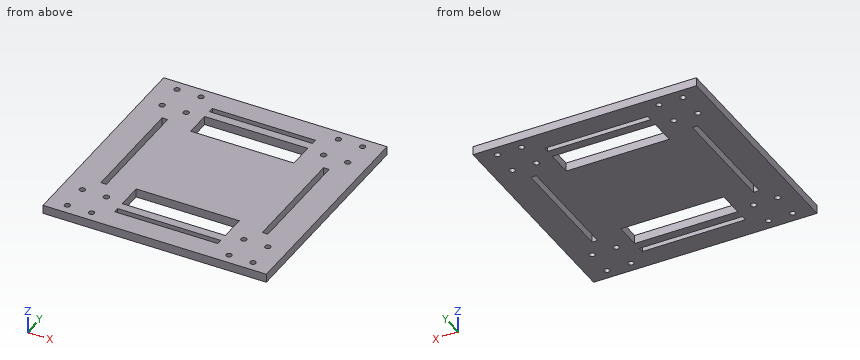
```python
from build123d import *

# Parameters (mm, degrees)
SKETCH_1_W          = 130
SKETCH_1_H          = 130
EXTRUDE_1_DEPTH     = 5
SKETCH_2_R          = 1.65
CUT_EXTRUDE_1_DEPTH = 5
SKETCH_3_W          = 3.2
SKETCH_3_H          = 66
SKETCH_3_W_2        = 60
SKETCH_3_H_2        = 3.2
CUT_EXTRUDE_2_DEPTH = 10
SKETCH_4_W          = 60
SKETCH_4_H          = 15
CUT_EXTRUDE_3_DEPTH = 10


with BuildPart() as part:
    # 草图1 → 凸台-拉伸1 (new body)
    with BuildSketch(Plane.XY):
        Rectangle(SKETCH_1_W, SKETCH_1_H)
    extrude(amount=EXTRUDE_1_DEPTH)

    # 草图2 → 切除-拉伸1 (cut)
    with BuildSketch(Plane.XY.offset(5)):
        with Locations((-54, 59)):
            Circle(SKETCH_2_R)
        with Locations((-40, 59)):
            Circle(SKETCH_2_R)
        with Locations((-40, 43)):
            Circle(SKETCH_2_R)
        with Locations((-54, 43)):
            Circle(SKETCH_2_R)
        with Locations((40, 59)):
            Circle(SKETCH_2_R)
        with Locations((54, 59)):
            Circle(SKETCH_2_R)
        with Locations((54, 43)):
            Circle(SKETCH_2_R)
        with Locations((40, 43)):
            Circle(SKETCH_2_R)
        with Locations((40, -43)):
            Circle(SKETCH_2_R)
        with Locations((54, -43)):
            Circle(SKETCH_2_R)
        with Locations((54, -59)):
            Circle(SKETCH_2_R)
        with Locations((40, -59)):
            Circle(SKETCH_2_R)
        with Locations((-54, -43)):
            Circle(SKETCH_2_R)
        with Locations((-40, -43)):
            Circle(SKETCH_2_R)
        with Locations((-40, -59)):
            Circle(SKETCH_2_R)
        with Locations((-54, -59)):
            Circle(SKETCH_2_R)
    extrude(amount=-CUT_EXTRUDE_1_DEPTH, mode=Mode.SUBTRACT)

    # 草图3 → 切除-拉伸2 (cut)
    with BuildSketch(Plane.XY.offset(5)):
        with Locations((47, 0)):
            Rectangle(SKETCH_3_W, SKETCH_3_H)
        with Locations((-47, 0)):
            Rectangle(SKETCH_3_W, SKETCH_3_H)
        with Locations((0, -51)):
            Rectangle(SKETCH_3_W_2, SKETCH_3_H_2)
        with Locations((0, 51)):
            Rectangle(SKETCH_3_W_2, SKETCH_3_H_2)
    extrude(amount=-CUT_EXTRUDE_2_DEPTH, mode=Mode.SUBTRACT)

    # 草图4 → 切除-拉伸3 (cut)
    with BuildSketch(Plane(origin=(0, 0, 0), x_dir=(-1, 0, 0), z_dir=(0, 0, -1))):
        with Locations((0, 36.9)):
            Rectangle(SKETCH_4_W, SKETCH_4_H)
        with Locations((0, -36.9)):
            Rectangle(SKETCH_4_W, SKETCH_4_H)
    extrude(amount=-CUT_EXTRUDE_3_DEPTH, mode=Mode.SUBTRACT)


solid = part.part
```
Read the model definition and answer for the solid it produces. Units are mm, in the model's axes. Coordinates: 2 decimals unless noted, no trailing zeros. Loops run counter-clockwise (first coordinate to the right, second up) from the corner with the lowest first, then second, coordinate; pieces in that order, holes last. Notation, with made-up numbers: (36.25, 84) -> (77.25, 84) arc R16 cw to (77.25, 115) -> close; hole circle Ø8 at (13.5, 84.25). An arc over 180 degrees is marked (long way). Return JSON: item names as keys, results as strings.
Item 1: Find section B-B (y = 6.5). Determine the outline of the cut face in (x, z).
Answers:
{"outline": "(-65, 0) -> (-48.6, 0) -> (-48.6, 5) -> (-65, 5) -> close; (-45.4, 0) -> (45.4, 0) -> (45.4, 5) -> (-45.4, 5) -> close; (48.6, 0) -> (65, 0) -> (65, 5) -> (48.6, 5) -> close"}
Item 2: Find the intervals of material crossed by probe 1 along X at (y, z) = (-7, 3.9); probe 2 along Y at (x, z) = (24, 2.3); probe 3 along X at (y, z) = (32, 0.45), in increasing order.
Answers:
{"probe 1": "x = -65 to -48.6, -45.4 to 45.4, 48.6 to 65", "probe 2": "y = -65 to -52.6, -49.4 to -44.4, -29.4 to 29.4, 44.4 to 49.4, 52.6 to 65", "probe 3": "x = -65 to -48.6, -45.4 to -30, 30 to 45.4, 48.6 to 65"}
Item 3: Find section A-A (y = 39.5). Determine the outline of the cut face in (x, z), plus the area to 3 significant figures.
Answers:
{"outline": "(-65, 0) -> (-30, 0) -> (-30, 5) -> (-65, 5) -> close; (30, 0) -> (65, 0) -> (65, 5) -> (30, 5) -> close", "area": "350 mm2"}
Item 4: Find section C-C (x = -40). Determine the outline of the cut face in (y, z).
Answers:
{"outline": "(-65, 0) -> (-60.65, 0) -> (-60.65, 5) -> (-65, 5) -> close; (-57.35, 0) -> (-44.65, 0) -> (-44.65, 5) -> (-57.35, 5) -> close; (-41.35, 0) -> (41.35, 0) -> (41.35, 5) -> (-41.35, 5) -> close; (44.65, 0) -> (57.35, 0) -> (57.35, 5) -> (44.65, 5) -> close; (60.65, 0) -> (65, 0) -> (65, 5) -> (60.65, 5) -> close"}
Item 5: Find section D-D (y = -59). Determine the outline of the cut face in (x, z), plus the area to 3 significant figures.
Answers:
{"outline": "(-65, 0) -> (-55.65, 0) -> (-55.65, 5) -> (-65, 5) -> close; (-52.35, 0) -> (-41.65, 0) -> (-41.65, 5) -> (-52.35, 5) -> close; (-38.35, 0) -> (38.35, 0) -> (38.35, 5) -> (-38.35, 5) -> close; (41.65, 0) -> (52.35, 0) -> (52.35, 5) -> (41.65, 5) -> close; (55.65, 0) -> (65, 0) -> (65, 5) -> (55.65, 5) -> close", "area": "584 mm2"}
Item 6: A flat-ended cylindrical pin translates along its axis: P1, Ø2.5, axis at x = -54, y = -43, coming from the -Z side. Find the tip coordinate at first contact, or state that the pin passes through.
Answers:
{"P1": "passes through"}
